Autodesk Inventor part; units mm, degrees
ref_plane "YZ Plane" through (0, 0, 0) normal (1, 0, 0) x (0, 1, 0)
ref_plane "XZ Plane" through (0, 0, 0) normal (0, 1, 0) x (-1, 0, 0)
ref_plane "XY Plane" through (0, 0, 0) normal (0, 0, 1) x (1, 0, 0)
sketch "Sketch1" plane through (0, 0, 0) normal (0, 1, 0) x (-1, 0, 0)
  line L0 (0, -5.4) -> (1.5, -5.4)
  line L1 (1.5, -5.4) -> (1.5, -8.1)
  line L2 (1.5, -8.1) -> (3.2, -8.1)
  line L3 (0, 0) -> (1.5, 0)
  line L4 (1.5, 0) -> (1.5, 2.7)
  line L5 (1.5, 2.7) -> (3.2, 2.7)
  line L6 (5, 0) -> (5, -5.4)
  line L7 (5, -5.4) -> (3.2, -8.1)
  line L8 (5, 0) -> (3.2, 2.7)
  line L9 (0, -5.4) -> (0, -12.7)
  line L10 (0, -12.7) -> (-5, -12.7)
  line L11 (-5, -12.7) -> (-5, 7.3)
  line L12 (-5, 7.3) -> (0, 7.3)
  line L13 (0, 7.3) -> (0, 0)
  dimension "d0" = 5.4
  dimension "d1" = 1.5
  dimension "d2" = 2.7
  dimension "d3" = 1.7
  dimension "d4" = 2.7
  dimension "d5" = 1.7
  dimension "d9" = 5
  dimension "d10" = 20
  dimension "d11" = 7.3
extrude "Extrusion1" add sketch "Sketch1" along normal blind 40
sketch "Sketch2" plane through (5, 0, 7.3) normal (1, 0, 0) x (0, 0, -1)
  line L0 (11.6599, 7.125) -> (8.3401, 7.125)
  line L1 (8.3401, 7.125) -> (6.6802, 10)
  line L2 (6.6802, 10) -> (8.3401, 12.875)
  line L3 (8.3401, 12.875) -> (11.6599, 12.875)
  line L4 (11.6599, 12.875) -> (13.3198, 10)
  line L5 (13.3198, 10) -> (11.6599, 7.125)
  line L6 (20, 0) -> (0, 0)
  line L7 (0, 0) -> (0, 40)
  line L8 (11.6599, 27.125) -> (8.3401, 27.125)
  line L9 (8.3401, 27.125) -> (6.6802, 30)
  line L10 (6.6802, 30) -> (8.3401, 32.875)
  line L11 (8.3401, 32.875) -> (11.6599, 32.875)
  line L12 (11.6599, 32.875) -> (13.3198, 30)
  line L13 (13.3198, 30) -> (11.6599, 27.125)
  line L14 (0, 40) -> (20, 40)
  point P0 (7.3, 0)
  point P1 (10, 10)
  point P2 (10, 30)
  dimension "d12" = 5.75
  dimension "d13" = 10
  dimension "d14" = 10
  dimension "d15" = 5.75
  dimension "d16" = 10
  dimension "d17" = 10
extrude "Extrusion2" cut sketch "Sketch2" against normal blind 2.5
sketch "Sketch3" plane through (2.5, 0, 7.3) normal (1, 0, 0) x (0, 0, -1)
  point P0 (7.3, 0)
sketch "Sketch4" plane through (2.5, 0, 7.3) normal (1, 0, 0) x (0, 0, -1)
  circle A0 centre (10, 10) radius 1.375
  circle A1 centre (10, 30) radius 1.375
  point P0 (7.3, 0)
  dimension "d20" = 2.75
  dimension "d21" = 2.75
extrude "Extrusion3" cut sketch "Sketch4" against normal blind 20
properties part number "slotMountingPlate"
The model under review builds one solid part; all positions refer to its coordinate system, in mm. A direction names the side the tool comes from. Coordinates: 2 decimals unless noted, no trailing zeros. Write each loop counter-clockwise with the first axis right and the second up, starting at its lowest first coordinate (ties: lowest second). Pieces come first, ordered by that corner, then holes.
1) We need section C-C on y = 15.5. State the section outline as (x, z) points, then the cut area to 3 significant figures.
2) We need section A-A on z = -2.7. State the section outline as (x, y) points (3 decimals).
3) We need section D-D on z = 1.5. State the section outline as (x, y) points, then the cut area to 3 significant figures.
4) We need section B-B on x = 4. State the section outline as (y, z) points (3 decimals).
5) Clearance check with flat-ended pins moving along their axes: pin 1 Ø1.6 at (x, y) = (-0.5, 24.5) entering from +Z; pin 2 Ø3.5 at (y, z) = (20.5, -9) entering from -X; pin 3 Ø2 at (y, z) = (27, 2) entering from -X; pin 4 Ø1.2 at (x, y) = (-1, 15.5) entering from -Z. State where each tip first meets the part, or that it passes through.
6) Machinability: for faces 5 (the face through (0, 20, 4)), 6 (the face through (-1, 20, -5.4)), 7 (the face through (3, 20, 7.3)), 8 (the face through (2.5, 11, -4)), 9 (the face through (-2, 20, 2.7)), which of the approach directions +Z, -Z, +X, -X, +Y, -Y give a long, thin tool a straight path to every point of the face, cutting with its end or side? Answer none if there is none.
7) To check wall thickness, follow probe 1 along Y at (x, z) = (1, -2.7) (3 decimals); probe 2 along Y at (x, z) = (4, -3.5) (3 decimals); probe 3 along X at (y, z) = (21.5, 3.75). State the ranges of each line that lie inside material, in increasing order.
8) The part is to be moulded in two halves that separate along X. For faces 1 (the face through (1, 40, -3)), 2 (the face through (5, 20, -3)), 3 (the face through (-1.5, 20, -7)), 4 (the face through (0, 20, -9)), say which applies: pulls with the +X half, pulls with the -X half, needs draft (parallel to the pull), parting line crosses it, or undercut.
Answer list:
1. outline: (-5, -5.4) - (-3.2, -8.1) - (-1.5, -8.1) - (-1.5, -5.4) - (0, -5.4) - (0, -12.7) - (5, -12.7) - (5, 7.3) - (0, 7.3) - (0, 0) - (-1.5, 0) - (-1.5, 2.7) - (-3.2, 2.7) - (-5, 0) - close
1. area: 141 mm2
2. outline: (-5, 0) - (5, 0) - (5, 7.125) - (2.5, 7.125) - (2.5, 8.625) - (-5, 8.625) - close; (-5, 11.375) - (2.5, 11.375) - (2.5, 12.875) - (5, 12.875) - (5, 27.125) - (2.5, 27.125) - (2.5, 28.625) - (-5, 28.625) - close; (-5, 31.375) - (2.5, 31.375) - (2.5, 32.875) - (5, 32.875) - (5, 40) - (-5, 40) - close
3. outline: (-4, 0) - (-1.5, 0) - (-1.5, 40) - (-4, 40) - close; (0, 0) - (5, 0) - (5, 40) - (0, 40) - close
3. area: 300 mm2
4. outline: (0, -12.7) - (40, -12.7) - (40, 7.3) - (0, 7.3) - close; hole (7.125, -4.36) - (10, -6.02) - (12.875, -4.36) - (12.875, -1.04) - (10, 0.62) - (7.125, -1.04) - close; hole (27.125, -4.36) - (30, -6.02) - (32.875, -4.36) - (32.875, -1.04) - (30, 0.62) - (27.125, -1.04) - close
5. pin 1: stops at z = 7.3
5. pin 2: stops at x = -3.77
5. pin 3: stops at x = -4.33
5. pin 4: stops at z = -8.1
6. face 5: +Z, +Y, -Y
6. face 6: -Z, +Y, -Y
6. face 7: +Z, +X, -X, +Y, -Y
6. face 8: +X
6. face 9: +Z, -X, +Y, -Y
7. probe 1: y = 0 to 8.625, 11.375 to 28.625, 31.375 to 40
7. probe 2: y = 0 to 7.125, 12.875 to 27.125, 32.875 to 40
7. probe 3: x = 0 to 5
8. face 1: needs draft
8. face 2: pulls with the +X half
8. face 3: undercut
8. face 4: undercut
